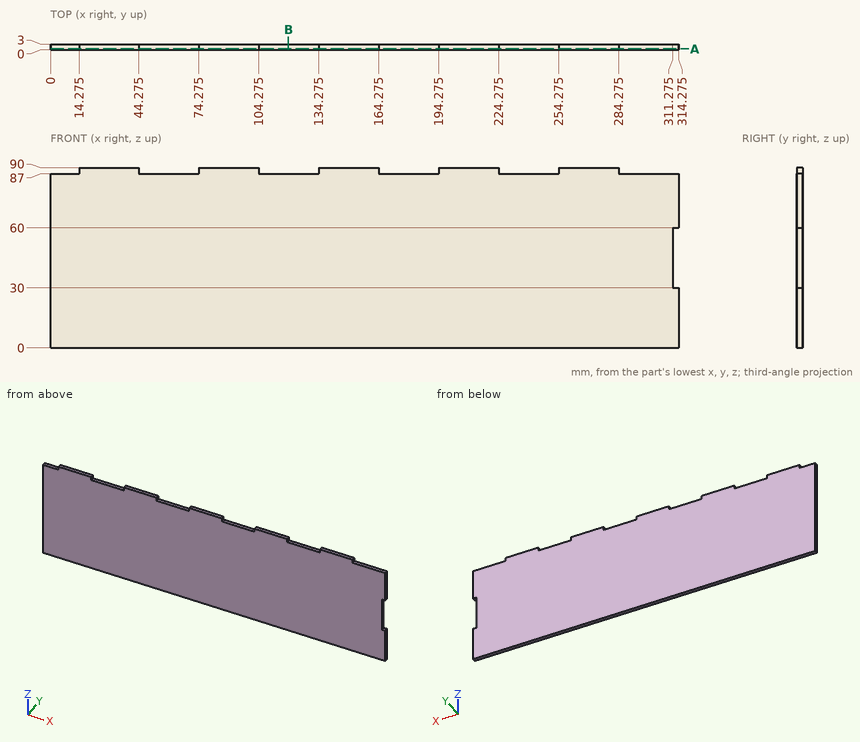
Geometry check sheet. Reference: drawing and pictorial views, mm from the part's lowest x, y, z. Coordinates: 2 decimals unless noted, no trailing zeros. Order: outer loops, then holes, each group sorted by start corner. A loop starts at its lowest first (then second) coordinate and runs counter-clockwise, first axis right, second up. Notation, with made-up numbers: M 87,36.25 L 106,36.25 A34 ccw 106,75.25 Z; hole C 32,-23 d8. An arc over 180 degrees is marked long. Return JSON: item names as keys, results as strings.
1) Gauge pin test, flat ends, axial feed: pin 1 (0.9 mm diameter, centred on x = 6, y = 2, fed in from +Z); pin 2 (1.5 mm diameter, centred on y = 1, z = 88, fed in from +X) (3 decimals); pin 3 (0.9 mm diameter, centred on y = 1, z = 89, fed in from -X) (3 decimals). Record the tip position at first contact, or that the pin passes through.
Answer list:
{"pin 1": "z = 87", "pin 2": "x = 284.275", "pin 3": "x = 14.275"}
2) Cross-section at A-A, the plane y = 0.55. Record the boundary of the cut face in (x, z) (3 decimals).
Answer list:
{"outline": "M 0,0 L 314.275,0 L 314.275,30 L 311.275,30 L 311.275,60 L 314.275,60 L 314.275,87 L 284.275,87 L 284.275,90 L 254.275,90 L 254.275,87 L 224.275,87 L 224.275,90 L 194.275,90 L 194.275,87 L 164.275,87 L 164.275,90 L 134.275,90 L 134.275,87 L 104.275,87 L 104.275,90 L 74.275,90 L 74.275,87 L 44.275,87 L 44.275,90 L 14.275,90 L 14.275,87 L 0,87 Z"}
3) Cross-section at B-B, the plane x = 119. Record the boundary of the cut face in (y, z), and give its area (3 significant figures).
Answer list:
{"outline": "M 0,0 L 3,0 L 3,87 L 0,87 Z", "area": "261 mm2"}
4) Thickness scan on L1, parallel to X at y = 1.1, z = 36 (3 decimals); L2, parallel to Z at x = 299.5, y = 2.75. Record the ranges inside material, lowest first. Write a range as [from, to].
Answer list:
{"L1": "[0, 311.275]", "L2": "[0, 87]"}
